```python
from build123d import *

# Parameters (mm, degrees)
F1_DEPTH = 15
F2_W     = 7.5
F2_H     = 12
F3_DEPTH = 20
F4_R     = 3.5
F5_DEPTH = 5


with BuildPart() as f1:
    # F0 (on Front) → F1 (new body, symmetric)
    with BuildSketch(Plane.XZ):
        Polygon((0, 42.711864), (0, 0), (0, -17.288136), (57.288132, -17.288136), (57.288132, -9.788136), (11.864405, -9.788136), (11.864405, 35.211864), (57.288132, 35.211864), (57.288132, 42.711864), align=None)
    extrude(amount=F1_DEPTH, both=True)

    # F2 (on face) → F3 (join)
    with BuildSketch(Plane.YZ.offset(11.864405)):
        with Locations((-0.309874, 12.711864)):
            Rectangle(F2_W, F2_H)
    extrude(amount=F3_DEPTH)

    # F4 (on face) → F5 (join)
    with BuildSketch(Plane.XZ.offset(4.059874)):
        with Locations((25.864405, 12.711864)):
            Circle(F4_R)
    extrude(amount=F5_DEPTH)


solid = f1.part
```
The model under review builds one solid part; all positions refer to its coordinate system, in mm. A direction names the side the tool comes from. Coordinates: 2 decimals unless noted, no trailing zeros. Order: outer loops, then holes, each group sorted by start corner. A loop starts at its lowest first (then second) coordinate and runs counter-clockwise, first axis right, second up. Notation, with made-up numbers: M -31.5,41 L 21.5,41 A12 ccw 21.5,54 Z; hole C 48,42 d11. An arc over 180 degrees is marked long. One line per question, with ' | ' between items.
(1) For probe 1 along Z at (x, y) = (19, -1.5); probe 2 along Z at (x, y) = (41, 4.5); probe 3 along X at (y, z) = (8, 1), list the stretches that pass through material, from the lowest coordinate up. Write a range as from..to.
Geometry results:
probe 1: z = -17.29..-9.79, 6.71..18.71, 35.21..42.71 | probe 2: z = -17.29..-9.79, 35.21..42.71 | probe 3: x = 0..11.86
(2) The part is to be moulded in two halves that separate along Z. For faces 4 (the face through (28, 0, -17.288)), 5 (the face through (22, -4.06, 13)), 6 (the face through (9, 15, 13)), say which applies: +Z half, -Z half, draft (parallel to the pull), parting line (faces both ways), or undercut.
Geometry results:
face 4: -Z half | face 5: undercut | face 6: draft
(3) Insertion check: pin 1 (1 mm diameter, centred on y = 5, z = -4.5, fed in from -X); pin 2 (3.5 mm diameter, centred on x = 26, z = 13, fed in from -Y); pin 3 (9.5 mm diameter, centred on x = 18.5, z = 10, fed in from +Y); pin 4 (4 mm diameter, centred on y = 7, z = 30, fed in from +X). Each pin has a flat end and moves straight along its axis. Give the tip position at first contact, or say it passes through.
Geometry results:
pin 1: stops at x = 0 | pin 2: stops at y = -9.06 | pin 3: stops at y = 3.44 | pin 4: stops at x = 11.86
(4) Add section A-A, the plane x = 53. Write out the cut boundary in (y, z).
Geometry results:
outline: M -15,-17.29 L 15,-17.29 L 15,-9.79 L -15,-9.79 Z; M -15,35.21 L 15,35.21 L 15,42.71 L -15,42.71 Z
(5) Add section B-B, the plane y = -13. Write out the cut boundary in (x, z).
Geometry results:
outline: M 0,-17.29 L 57.29,-17.29 L 57.29,-9.79 L 11.86,-9.79 L 11.86,35.21 L 57.29,35.21 L 57.29,42.71 L 0,42.71 Z
(6) Add section C-C, the plane x = 16. Write out the cut boundary in (y, z).
Geometry results:
outline: M -15,-17.29 L 15,-17.29 L 15,-9.79 L -15,-9.79 Z; M -15,35.21 L 15,35.21 L 15,42.71 L -15,42.71 Z; M -4.06,6.71 L 3.44,6.71 L 3.44,18.71 L -4.06,18.71 Z
(7) Add section D-D, the plane y = -5.5. Write out the cut boundary in (x, z), then the cut area to 3 significant figures.
Geometry results:
outline: M 0,-17.29 L 57.29,-17.29 L 57.29,-9.79 L 11.86,-9.79 L 11.86,35.21 L 57.29,35.21 L 57.29,42.71 L 0,42.71 Z; C 25.86,12.71 d7 | area: 1,430 mm²
(8) Machinability: for faces 1 (the face through (29.203, -6.525, 13.763)), 2 (the face through (22, 3.44, 13)), 3 (the face through (22, 0, 6.712)), which of the approach directions +Z, -Z, +X, -X, +Y, -Y give a long, thin tool a straight path to every point of the face, cutting with its end or side? Answer none if there is none.
Geometry results:
face 1: -Y | face 2: +X, +Y | face 3: +X, +Y, -Y
